from build123d import *

# Parameters (mm, degrees)
SKETCH1_R           = 3.3655
SKETCH1_R_2         = 2.5
BOSS_EXTRUDE1_DEPTH = 2.54
SKETCH2_R           = 1.143
SKETCH2_R_2         = 0.6604
SKETCH2_R_3         = 1.5
BOSS_EXTRUDE2_DEPTH = 1.7272
FILLET1_R           = 12.7
CUT_EXTRUDE1_START  = -1.27
SKETCH3_R           = 2.06375
SKETCH3_R_2         = 1.143
CUT_EXTRUDE1_DEPTH  = 1.27


with BuildPart() as part:
    # Sketch1 → Boss-Extrude1 (new body)
    with BuildSketch(Plane(origin=(0, 0, 0), x_dir=(1, 0, 0), z_dir=(0, 1, 0))):
        with Locations(Location((0, 0, 0), (0, 0, 270))):
            Circle(SKETCH1_R)
        with Locations(Location((0, 0, 0), (0, 0, 270))):
            Circle(SKETCH1_R_2, mode=Mode.SUBTRACT)
    extrude(amount=BOSS_EXTRUDE1_DEPTH)

    # Sketch2 → Boss-Extrude2 (add)
    with BuildSketch(Plane(origin=(0, 2.54, 0), x_dir=(1, 0, 0), z_dir=(0, 1, 0))):
        with BuildLine():
            Line((0, 3.8227), (-16.092265178, 2.307544345))
            ThreePointArc((-16.092265178, 2.307544345), (-18.19275, 0), (-16.092265178, -2.307544345))
            Line((-16.092265178, -2.307544345), (0, -3.8227))
            Line((0, -3.8227), (16.092265178, -2.307544345))
            ThreePointArc((16.092265178, -2.307544345), (18.19275, 0), (16.092265178, 2.307544345))
            Line((16.092265178, 2.307544345), (0, 3.8227))
        make_face()
        with BuildLine():
            ThreePointArc((9.8806, -1.5), (8.3806, 0), (9.8806, 1.5))
            Line((9.8806, 1.5), (15.875, 1.5))
            ThreePointArc((15.875, 1.5), (17.375, 0), (15.875, -1.5))
            Line((15.875, -1.5), (9.8806, -1.5))
        make_face(mode=Mode.SUBTRACT)
        with Locations(Location((0, 0, 0), (0, 0, 270))):
            Circle(SKETCH2_R, mode=Mode.SUBTRACT)
        with Locations(Location((7.1628, 0, 0), (0, 0, 270))):
            Circle(SKETCH2_R_2, mode=Mode.SUBTRACT)
        with Locations(Location((-7.1628, 0, 0), (0, 0, 270))):
            Circle(SKETCH2_R_2, mode=Mode.SUBTRACT)
        with Locations(Location((-12.8778, 0, 0), (0, 0, 270))):
            Circle(SKETCH2_R_2, mode=Mode.SUBTRACT)
        with Locations(Location((-9.8806, 0, 0), (0, 0, 270))):
            Circle(SKETCH2_R_2, mode=Mode.SUBTRACT)
        with Locations(Location((-15.875, 0, 0), (0, 0, 270))):
            Circle(SKETCH2_R_3, mode=Mode.SUBTRACT)
    extrude(amount=BOSS_EXTRUDE2_DEPTH)

    # Fillet1
    fillet1_edges = [part.edges().sort_by_distance(p)[0] for p in [
        (0, 3.4036, 3.8227),
        (0, 3.4036, -3.8227),
    ]]
    fillet(fillet1_edges, radius=FILLET1_R)

    # Sketch3 → Cut-Extrude1 (cut)
    with BuildSketch(Plane(origin=(0, 4.2672, 0), x_dir=(1, 0, 0), z_dir=(0, 1, 0)).offset(CUT_EXTRUDE1_START)):
        with Locations(Location((0, 0, 0), (0, 0, 270))):
            Circle(SKETCH3_R)
        with Locations(Location((0, 0, 0), (0, 0, 270))):
            Circle(SKETCH3_R_2, mode=Mode.SUBTRACT)
    extrude(amount=CUT_EXTRUDE1_DEPTH, mode=Mode.SUBTRACT)


solid = part.part
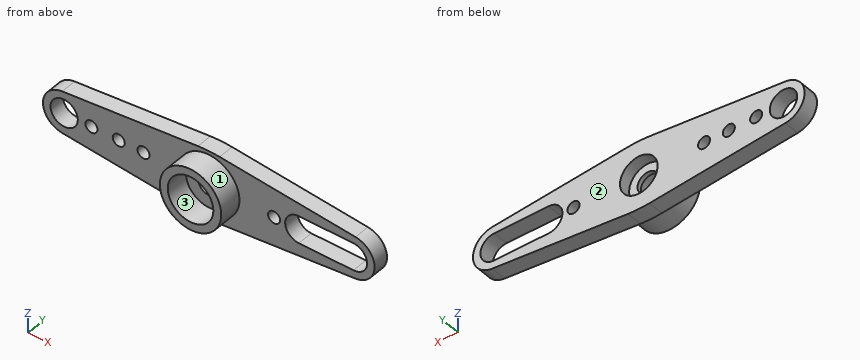
Work out the finished part from the listing and answer in its coordinate system (mm). Face numbers are marked on the shaded views. Give positions to 0.01 mm unless a question says otherwise; leave off trailing zeros. Order: outer loops, then holes, each group sorted by start corner. A loop starts at its lowest first (then second) coordinate and runs counter-clockwise, first axis right, second up. Notation, with made-up numbers: M -37,-12 L 19,-12 A15 ccw 19,1 Z; hole C -30,74.25 d6. An arc over 180 degrees is marked long. Return JSON: item names as keys, results as strings.
Q1. Find the intervals of material crossed by line 1 along X through (y, z) = (0.7, 0); line 2 along X through (y, z) = (3.65, -0.75); line 3 along Y through (x, z) = (8, -0.5), in increasing order. Write a range as [from, to].
Answer below:
{"line 1": "x = [-3.37, -2.5], [2.5, 3.37]", "line 2": "x = [-18.07, -17.17], [-14.58, -1.92], [1.92, 8.58], [17.17, 18.07]", "line 3": "y = [2.54, 4.27]"}
Q2. Find section C-C, the plane y = 1.9. Write down the section's boundary in (x, z).
Answer below:
{"outline": "C 0,0 d6.73; hole C 0,0 d5"}
Q3. The mould has two halves that part along X. Classify the marked faces 1, 2 and 3: pulls with the +X half, pulls with the -X half, needs draft (parallel to the pull), parting line crosses it, or undercut.
Answer below:
{"face 1": "parting line crosses it", "face 2": "needs draft", "face 3": "undercut"}
Q4. Find section D-D, the plane x = -15. Write down the section's boundary in (y, z), and give its area (3 significant figures).
Answer below:
{"outline": "M 2.54,-2.41 L 4.27,-2.41 L 4.27,-1.22 L 2.54,-1.22 Z; M 2.54,1.22 L 4.27,1.22 L 4.27,2.41 L 2.54,2.41 Z", "area": "4.12 mm^2"}
Q5. Find section A-A, the plane x = 0. Write down the section's boundary in (y, z), and give its area (3 significant figures).
Answer below:
{"outline": "M 0,-3.37 L 2.54,-3.37 L 2.54,-3.77 L 4.27,-3.77 L 4.27,-2.06 L 3,-2.06 L 3,-1.14 L 2.54,-1.14 L 2.54,-2.5 L 0,-2.5 Z; M 0,2.5 L 2.54,2.5 L 2.54,1.14 L 3,1.14 L 3,2.06 L 4.27,2.06 L 4.27,3.77 L 2.54,3.77 L 2.54,3.37 L 0,3.37 Z", "area": "11.1 mm^2"}
Q6. Find section B-B, the plane z = 0. State how many separate pieces and enclosed holes the cut face has, and give its area (3 significant figures).
Answer below:
{"separate pieces": "8", "enclosed holes": "0", "area": "31.1 mm^2"}
Q7. Each of these flat-tipped pins is pushed along its axis until it touches: pin 1 (1.7 mm diameter, centred on x = -12.88, z = 0, fed in from -Y); pin 2 (1.4 mm diameter, centred on x = 13, y = 3.5, fed in from -Z); pin 3 (1.5 mm diameter, centred on y = 3.5, z = 2.5, fed in from +X). Where does it stop, or does it pass through?
Answer below:
{"pin 1": "stops at y = 2.54", "pin 2": "stops at z = -2.66", "pin 3": "stops at x = 17.39"}
